Design review of the part built by this model. Coordinates are the model's own, in mm. A direction names the side the tool comes from. Coordinates: 2 decimals unless noted, no trailing zeros. Loops run counter-clockwise (first coordinate to the right, second up) from the corner with the lowest first, then second, coordinate; pieces in that order, holes last. Notation, with made-up numbers: M 57,-3.5 L 85,-3.5 A15 ccw 85,20.5 Z; hole C 87,32.5 d7. An arc over 180 degrees is marked long. Answer as CSV lines item,"result". Start each with the question number.
from build123d import *

# Parameters (mm, degrees)
SKETCH1_W           = 23.75
SKETCH1_H           = 24
BOSS_EXTRUDE1_DEPTH = 10
SKETCH2_W           = 3.3
SKETCH2_H           = 9.8
BOSS_EXTRUDE2_DEPTH = 23.75
CUT_EXTRUDE1_REACH  = 36.413
SKETCH4_R           = 1.9
SKETCH5_W           = 3.5
SKETCH5_H           = 3.25
SKETCH5_H_2         = 17.5
SKETCH5_W_2         = 3.3
SKETCH5_H_3         = 9.8
CUT_EXTRUDE2_DEPTH  = 5


with BuildPart() as part:
    # Sketch1 → Boss-Extrude1 (new body)
    with BuildSketch(Plane.YZ):
        with Locations((11.875, 12)):
            Rectangle(SKETCH1_W, SKETCH1_H)
    extrude(amount=-BOSS_EXTRUDE1_DEPTH)

    # Sketch2 → Boss-Extrude2 (add, through all)
    with BuildSketch(Plane.XZ):
        with Locations((-5, -4.9)):
            Rectangle(SKETCH2_W, SKETCH2_H)
    extrude(amount=-BOSS_EXTRUDE2_DEPTH)

    # Sketch4 → Cut-Extrude1 (cut, up to next)
    with BuildSketch(Plane(origin=(-6.65, 0, 0), x_dir=(0, -1, 0), z_dir=(-1, 0, 0)), mode=Mode.PRIVATE) as cut_extrude1_sk1:
        with Locations(Location((-11.875, -5, 0), (0, 0, 90))):
            Circle(SKETCH4_R)
    cut_extrude1_tool1 = extrude(cut_extrude1_sk1.sketch, amount=-CUT_EXTRUDE1_REACH, mode=Mode.PRIVATE) & part.part
    add(cut_extrude1_tool1.solids().sort_by_distance((-6.65, 11.875, -5))[0], mode=Mode.SUBTRACT)

    # Sketch5 → Cut-Extrude2 (cut)
    with BuildSketch(Plane(origin=(0, 23.75, 0), x_dir=(-1, 0, 0), z_dir=(0, 1, 0))):
        with Locations((5, 22.375)):
            Rectangle(SKETCH5_W, SKETCH5_H)
        with Locations((5, 12)):
            Rectangle(SKETCH5_W, SKETCH5_H_2)
        Polygon((6.75, 3.25), (3.25, 3.25), (3.25, 0), (3.35, 0), (6.65, 0), (6.75, 0), align=None)
        with Locations((5, -4.9)):
            Rectangle(SKETCH5_W_2, SKETCH5_H_3)
    cut_extrude2 = extrude(amount=-CUT_EXTRUDE2_DEPTH, mode=Mode.SUBTRACT)

    # Mirror1: Cut-Extrude2 across plane
    add(cut_extrude2.mirror(Plane.ZX.offset(11.875)), mode=Mode.SUBTRACT)


solid = part.part
Item 1: Add section D-D (x = -7.5). Give the boundary of the cut face in (y, z).
Item 2: For faces 4 (the face through (-2, 12, 0)), 5 (the face through (-8, 12, 0)), 6 (the face through (-5, 5, 7)), 7 (the face through (-3.25, 21, 12)), 8 (the face through (-10, 12, 12)), list the 3-axis set-ups (+Z, -Z, +X, -X, +Y, -Y) from which the entire face can be reached by the end or side of a thin tool; tool diameter is ignored.
Item 3: For pin 1 (3 mm diameter, centred on y = 11.875, z = -5, fed in from +X); pin 2 (3.5 mm diameter, centred on x = -1.5, y = 14.5, fed in from -Z); pin 3 (5 mm diameter, centred on y = 8.5, z = -6, fed in from +X), all flat-tipped, find the tip position at first contact; note any pin that passes through.
Item 4: Add section A-A (z = -5). Give the boundary of the cut face in (x, y) (3 decimals).
Item 5: For line 1 along Y through (x, z) = (-4.85, -5) (3 decimals); line 2 along Z through (x, y) = (-5.25, 12); line 3 along X through (y, z) = (20, 18), list the stretches that pass through material, from the lowest coordinate up. Write a range as from..to.
Item 6: Mouldability with a two-part tool opening along Y and no side actions: class faces 1 (the face through (-5.02, 11.96, -6.9)), 2 (the face through (-8, 23.75, 12)), 3 (the face through (-6.75, 21, 12)) as released by +Y, released by -Y, zero draft, split by the parting line, or undercut.
Item 7: Add section B-B (z = 6). Give the boundary of the cut face in (x, y), plus the area to 4 significant figures.
Item 8: Add section C-C (y = 8.5). Give the boundary of the cut face in (x, z), plus the area to 3 significant figures.
Response:
1,outline,"M 0,0 L 23.75,0 L 23.75,24 L 0,24 Z"
2,face 4,"-Z, +X, +Y, -Y"
2,face 5,"-Z, -X, +Y, -Y"
2,face 6,"+Z, -Z, -Y"
2,face 7,"+Z, -Z, +Y"
2,face 8,"+Z, -Z, -X, +Y, -Y"
3,pin 1,"through"
3,pin 2,"z = 0"
3,pin 3,"x = -3.35"
4,outline,"M -6.65,5 L -3.35,5 L -3.35,9.975 L -6.65,9.975 Z; M -6.65,13.775 L -3.35,13.775 L -3.35,18.75 L -6.65,18.75 Z"
5,line 1,"5..9.975, 13.775..18.75"
5,line 2,"-9.8..-6.9, -3.1..24"
5,line 3,"-10..-6.75, -3.25..0"
6,face 1,"undercut"
6,face 2,"released by +Y"
6,face 3,"zero draft"
7,outline,"M -10,0 L -6.75,0 L -6.75,5 L -3.25,5 L -3.25,0 L 0,0 L 0,23.75 L -3.25,23.75 L -3.25,18.75 L -6.75,18.75 L -6.75,23.75 L -10,23.75 Z"
7,area,"202.5 mm²"
8,outline,"M -10,0 L -6.65,0 L -6.65,-9.8 L -3.35,-9.8 L -3.35,0 L 0,0 L 0,24 L -10,24 Z"
8,area,"272 mm²"
